from build123d import *

# Parameters (mm, degrees)
SKETCH1_R           = 48.73625
BOSS_EXTRUDE1_DEPTH = 177.8
DOME1_FACE_RADIUS   = 48.73625
DOME1_HEIGHT        = 49.2125
DOME2_FACE_RADIUS   = 48.73625
DOME2_HEIGHT        = 49.2125


with BuildPart() as part:
    # Sketch1 → Boss-Extrude1 (new body)
    with BuildSketch(Plane.XY):
        Circle(SKETCH1_R)
    extrude(amount=BOSS_EXTRUDE1_DEPTH)

    # Dome1: a dome of height H over a round flat face of radius A is a cap of a sphere of radius (A * A + H * H) / (2 * H)
    dome1_r = (DOME1_FACE_RADIUS * DOME1_FACE_RADIUS + DOME1_HEIGHT * DOME1_HEIGHT) / (2 * DOME1_HEIGHT)
    dome1_base = Plane((0, 0, 177.8), z_dir=(0, 0, 1))
    with Locations(dome1_base.offset(DOME1_HEIGHT - dome1_r)):
        dome1_ball = Sphere(dome1_r, mode=Mode.PRIVATE)
    add(split(dome1_ball, bisect_by=dome1_base, keep=Keep.TOP, mode=Mode.PRIVATE))

    # Dome2: a dome of height H over a round flat face of radius A is a cap of a sphere of radius (A * A + H * H) / (2 * H)
    dome2_r = (DOME2_FACE_RADIUS * DOME2_FACE_RADIUS + DOME2_HEIGHT * DOME2_HEIGHT) / (2 * DOME2_HEIGHT)
    dome2_base = Plane((0, 0, 0), z_dir=(0, 0, -1))
    with Locations(dome2_base.offset(DOME2_HEIGHT - dome2_r)):
        dome2_ball = Sphere(dome2_r, mode=Mode.PRIVATE)
    add(split(dome2_ball, bisect_by=dome2_base, keep=Keep.TOP, mode=Mode.PRIVATE))


solid = part.part
CAD build for the part. Positions are in the model's coordinates, mm. Coordinates: 2 decimals unless noted, no trailing zeros. Loops run counter-clockwise (first coordinate to the right, second up) from the corner with the lowest first, then second, coordinate; pieces in that order, holes last. Notation, with made-up numbers: (14, 2) - (54, 2) arc R19 ccw to (54, 9) - close; hole circle Ø10 at (77, -5.5). An arc over 180 degrees is marked (long way). Write item = value, one per line. Start each with the question number.
Q1. Cut at D-D, the plane z = 181. List the corners of the cut face in (x, y).
Q2. Cut at C-C, the plane z = 97. List the corners of the cut face in (x, y), then the cut area to 3 significant figures.
Q3. Drill centre lines: L1, parallel to X at y = -1, z = 10; L2, parallel to Y at x = 18.5, z = 96.5; L3, parallel to X at y = -27, z = 103.5. Where is each one in solid material? Low to high.
Q4. Flat gauge pins, fed straight in: pin 1 Ø5 at (y, z) = (-1, -8) entering from -X; pin 2 Ø3 at (x, y) = (8.5, -22) entering from -Z; pin 3 Ø1.5 at (y, z) = (-2.5, 158.5) entering from +X. Where does each tip first touch, or does it go through?
Computed:
q1.outline = circle Ø97.32 at (0, 0)
q2.outline = circle Ø97.47 at (0, 0)
q2.area = 7,460 mm²
q3.L1 = -48.73 to 48.73
q3.L2 = -45.09 to 45.09
q3.L3 = -40.57 to 40.57
q4.pin_1 = -48.47
q4.pin_2 = -43.92
q4.pin_3 = 48.7
